Part print with two shaded views. Sizes in mm from the minimum x, y, z corner. Coordinates: 2 decimals unless noted, no trailing zeros. Loops run counter-clockwise (first coordinate to the right, second up) from the corner with the lowest first, then second, coordinate; pieces in that order, holes last.
Item 1: Cut at A-A (x = 68.37). List the corners of the cut face in (y, z).
Item 2: Cut at D-D (x = 103). List the corners of the cut face in (y, z), and give its area (3 significant figures).
Item 3: Drill centre lines: line 1 along X through (y, z) = (0.3, 68.37); line 2 along Z through (x, y) = (38.5, 0.2) (1 decimal). Where is each one in solid material? Low to high.
Item 4: Flat gauge pin, fed straight in: pin 1 (11.5 mm diameter, centred on x = 36.89, z = 100.52, fed in from +Y). Where does the tip first touch, or does it go through?
Item 5: Cut at C-C (y = 0.75). List the corners of the cut face in (x, z) (1 decimal), and give its area (3 significant figures).
Item 6: Cut at B-B (z = 41). List the corners of the cut face in (x, y) (1 decimal), and give its area (3 significant figures).
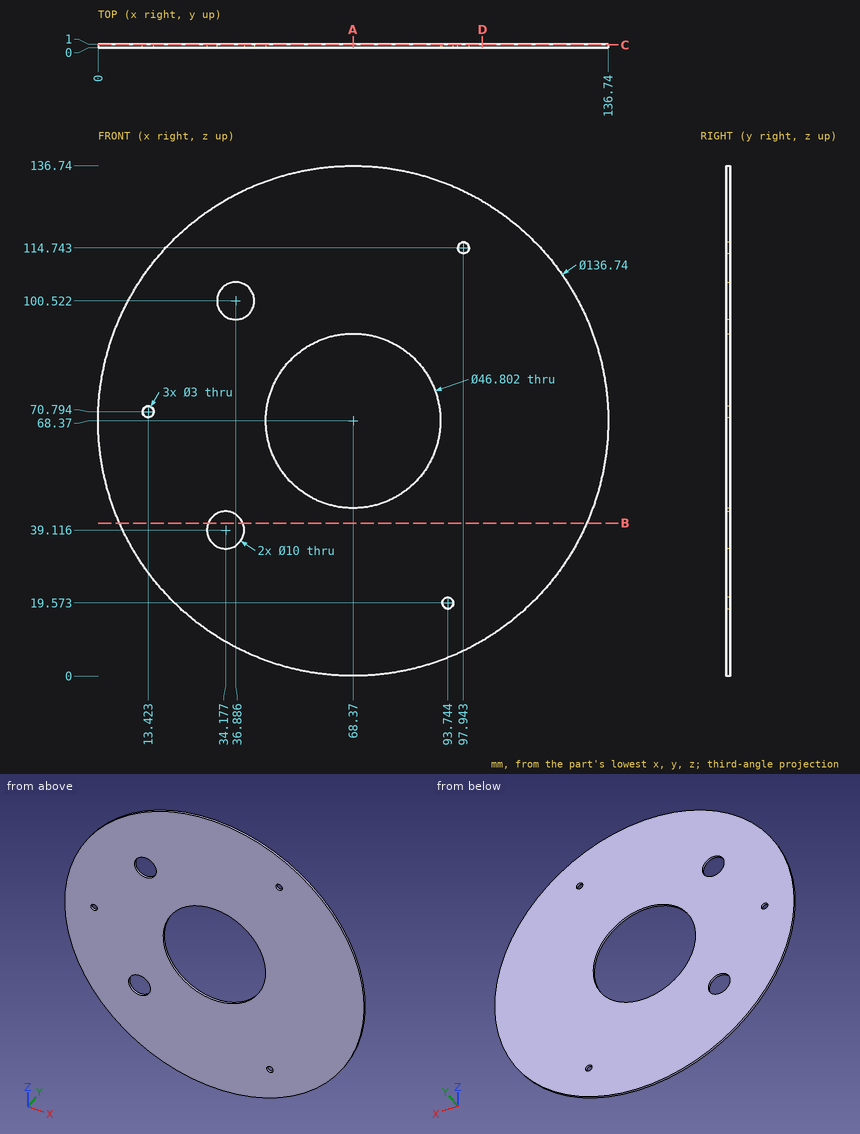
Filled sheet:
1. outline: (0, 0) - (1, 0) - (1, 44.97) - (0, 44.97) - close; (0, 91.77) - (1, 91.77) - (1, 136.74) - (0, 136.74) - close
2. outline: (0, 9.42) - (1, 9.42) - (1, 127.32) - (0, 127.32) - close
2. area: 118 mm2
3. line 1: x = 0 to 44.97, 91.77 to 136.74
3. line 2: z = 6.9 to 36.6, 41.6 to 95.8, 105.3 to 129.9
4. pin 1: stops at y = 1
5. outline: circle Ø136.7 at (68.4, 68.4); hole circle Ø3 at (13.4, 70.8); hole circle Ø10 at (34.2, 39.1); hole circle Ø10 at (36.9, 100.5); hole circle Ø46.8 at (68.4, 68.4); hole circle Ø3 at (93.7, 19.6); hole circle Ø3 at (97.9, 114.7)
5. area: 12,800 mm2
6. outline: (5.7, 0) - (29.5, 0) - (29.5, 1) - (5.7, 1) - close; (38.8, 0) - (131, 0) - (131, 1) - (38.8, 1) - close
6. area: 116 mm2
